Can you work these out from the model? Positions are in its coordinate system, mm. Face numbers are marked on the shaded views. A direction names the side the tool comes from. Round coordinates to 2 decimals unless told otherwise and drop trailing zeros. Write each loop counter-clockwise with the first axis right and the second up, starting at its lowest first coordinate (ties: lowest second). Pieces come first, ordered by that corner, then holes. Notation, with made-up numbers: (73, -13.75) - (110, -13.75) arc R33 cw to (110, 20.25) - close; hole circle Ø4 at (-2.5, 13.5). An arc over 180 degrees is marked (long way). One line per item, written item: value. Start each with the question number.
(1) I want a section at A-A on z = -35. List the corners of the cut face in (x, y) for me (3 decimals).
(2) If I drill on L1, parallel to X at y = -6.85, z = -35 (3 decimals); L2, parallel to X at y = -8.75, z = -32; L3, parallel to Z at x = -17.5, y = -5, over which ranges is the centre line in solid material (lowest first)? Write a range as from..to.
(3) I'm going to push flat-ended pins straight in: pin 1 Ø8 at (x, z) = (11, -121.5) entering from +Y; pin 2 Ø2 at (x, y) = (-6.5, -1.5) entering from -Z; pin 3 Ø10 at (y, z) = (-3.5, -134.5) entering from -X; pin 4 Ø11 at (x, z) = (1, -119) entering from -Y. Where does each tip first touch, or does it pass through?
(4) I want a section at B-B on z = -49.95. List the corners of the cut face in (x, y) for me.
(5) I want a section at C-C on z = -95. List the corners of the cut face in (x, y) for me (3 decimals), plus the area to 3 significant figures.
(6) I want a section at D-D on x = 2. List the corners of the cut face in (y, z) for me.
(7) On a 3-axis mill with a long thin cutter (end or side, diameter ignored), from which of +Z, -Z, +X, -X, +Y, -Y can I reach the whole of each face in a straight line? I mean the marked faces 4 and 5. Say none if no direction works.
(8) Thinking about a two-plate mould opening in X: for the marked faces 1, 2 and 3, which applies, +X half, -X half, draft (parallel to the pull), parting line (faces both ways), or undercut?
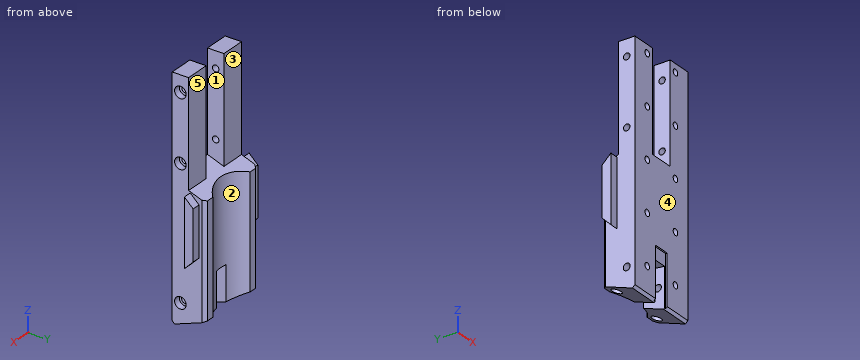
from build123d import *

# Parameters (mm, degrees)
SKETCH_1_W               = 63.621503831
SKETCH_1_H               = 9.95
EXTRUDE_1_DEPTH          = 22.5
CUT_EXTRUDE_START        = -7.55
CUT_EXTRUDE_1_DEPTH      = 15.1
CUT_EXTRUDE_2_DEPTH      = 145.249434495
CUT_EXTRUDE_2_DEPTH_BACK = 145.249434495
SKETCH_2_R               = 1.95
EXTRUDE_3_DEPTH          = 27.5
CUT_EXTRUDE_6_DEPTH      = 4.05
SKETCH_3_R               = 22.6
CUT_EXTRUDE_3_DEPTH      = 146.113401697
CUT_EXTRUDE_7_DEPTH      = 146.113401697
CUT_EXTRUDE_7_DEPTH_BACK = 146.113401697
SKETCH_10_R              = 2.1
SKETCH_11_W              = 39.483635772
SKETCH_11_H              = 6.923947262
CUT_EXTRUDE_8_DEPTH      = 5
CHAMFER_1_SIZE           = 2
SKETCH_4_R               = 3.5
CUT_EXTRUDE_4_DEPTH      = 4
SKETCH_12_R              = 3
CUT_EXTRUDE_9_DEPTH      = 3.1
CHAMFER_2_SIZE           = 2
CHAMFER_2_SIZE2          = 1.560412017
CHAMFER_2_EDGE_2_SIZE    = 2
CHAMFER_2_EDGE_2_SIZE2   = 1.560412017
SKETCH_13_R              = 1.925
CUT_EXTRUDE_10_DEPTH     = 5


# Read off the part's stored shape, not the designer's step: 컷-돌출1
with BuildPart() as part:
    # 스케치1 → 보스-돌출1 (new, symmetric)
    with BuildSketch(Plane(origin=(0, 0, 0), x_dir=(0, 0, -1), z_dir=(1, 0, 0))):
        with Locations((31.810751916, -4.975)):
            Rectangle(SKETCH_1_W, SKETCH_1_H)
        Polygon((142.136015324, -9.95), (63.621503831, -9.95), (63.621503831, 0), (67.243007662, 9.95), (134.893007662, 9.95), align=None)
        Polygon((63.621503831, -9.95), (63.621503831, 0), (60, -9.95), align=None)
    extrude(amount=EXTRUDE_1_DEPTH, both=True)

    # 컷-돌출1 outline → 컷-돌출1 (cut)
    with BuildSketch(Plane(origin=(0, 0, 0), x_dir=(0, 0, -1), z_dir=(1, 0, 0)).offset(CUT_EXTRUDE_START)):
        Polygon((60, -9.95), (63.621503831, 0), (0, 0), (0, -9.95), align=None)
    extrude(amount=CUT_EXTRUDE_1_DEPTH, mode=Mode.SUBTRACT)

    # 스케치2 → 컷-돌출2 (cut, two sides: drawn at the far end of the back side and taken through both)
    with BuildSketch(Plane(origin=(0, 0, 0), x_dir=(0, 0, -1), z_dir=(1, 0, 0)).offset(-CUT_EXTRUDE_2_DEPTH_BACK)):
        with Locations((9.95, -5)):
            Circle(SKETCH_2_R)
        with Locations((49.95, -5)):
            Circle(SKETCH_2_R)
    extrude(amount=CUT_EXTRUDE_2_DEPTH + CUT_EXTRUDE_2_DEPTH_BACK, mode=Mode.SUBTRACT)

    # 스케치6 → 보스-돌출3 (add, symmetric)
    with BuildSketch(Plane(origin=(0, 0, 0), x_dir=(0, 0, -1), z_dir=(1, 0, 0))):
        Polygon((64.701480994, 1.014614629), (69.728626839, 6.30205348), (99.728626839, 6.30205348), (105.104415209, 1.014614629), align=None)
    extrude(amount=EXTRUDE_3_DEPTH, both=True)

    # 스케치9 → 컷-돌출6 (cut, symmetric)
    with BuildSketch(Plane(origin=(0, 0, 0), x_dir=(0, 0, -1), z_dir=(1, 0, 0))):
        Polygon((139.292204442, 9.95), (148.391731499, -9.95), (117.656886036, -9.95), (115.43958996, 9.95), align=None)
    extrude(amount=CUT_EXTRUDE_6_DEPTH, both=True, mode=Mode.SUBTRACT)

    # 스케치3 → 컷-돌출3 (cut, through all)
    with BuildSketch(Plane.XY):
        with Locations((0, 26)):
            Circle(SKETCH_3_R)
    extrude(amount=-CUT_EXTRUDE_3_DEPTH, mode=Mode.SUBTRACT)

    # 스케치10 → 컷-돌출7 (cut, two sides: drawn at the far end of the back side and taken through both)
    with BuildSketch(Plane(origin=(0, 0, 0), x_dir=(0, 0, -1), z_dir=(1, 0, 0)).offset(-CUT_EXTRUDE_7_DEPTH_BACK)):
        with Locations((128.602443504, -5)):
            Circle(SKETCH_10_R)
    extrude(amount=CUT_EXTRUDE_7_DEPTH + CUT_EXTRUDE_7_DEPTH_BACK, mode=Mode.SUBTRACT)

    # 스케치11 → 컷-돌출8 (cut, symmetric)
    with BuildSketch(Plane(origin=(0, 0, 0), x_dir=(0, 0, -1), z_dir=(1, 0, 0))):
        with Locations((129.741817886, -12.461973631)):
            Rectangle(SKETCH_11_W, SKETCH_11_H)
    extrude(amount=CUT_EXTRUDE_8_DEPTH, both=True, mode=Mode.SUBTRACT)

    # 모따기1
    chamfer_1_edges = [part.edges().sort_by_distance(p)[0] for p in [
        (22.5, 9.95, -101.068007662),
        (-22.5, 9.95, -101.068007662),
    ]]
    chamfer(chamfer_1_edges, length=CHAMFER_1_SIZE)

    # 스케치4 → 컷-돌출4 (cut)
    with BuildSketch(Plane(origin=(22.5, 0, 0), x_dir=(0, 0, -1), z_dir=(1, 0, 0))):
        with Locations((9.95, -5)):
            Circle(SKETCH_4_R)
        with Locations((49.95, -5)):
            Circle(SKETCH_4_R)
        with Locations((128.602443504, -5)):
            Circle(SKETCH_4_R)
    extrude(amount=-CUT_EXTRUDE_4_DEPTH, mode=Mode.SUBTRACT)

    # 스케치12 → 컷-돌출9 (cut)
    with BuildSketch(Plane(origin=(0, 44.517705875, -122.311391657), x_dir=(-1, 0, 0), z_dir=(0, 0.3420201433256732, -0.9396926207859068))):
        with Locations(Location((-17, -42, 0), (0, 0, 90))):
            Circle(SKETCH_12_R)
        with Locations(Location((17, -42, 0), (0, 0, 90))):
            Circle(SKETCH_12_R)
    extrude(amount=-CUT_EXTRUDE_9_DEPTH, mode=Mode.SUBTRACT)

    # 모따기2
    chamfer_2_edges = [part.edges().sort_by_distance(p)[0] for p in [
        (-13.75, -9.95, -142.136015324),
    ]]
    chamfer_2_side = [part.faces().sort_by_distance(p)[0] for p in [
        (0, -9.95, -74.847019357),
    ]]
    chamfer(chamfer_2_edges, length=CHAMFER_2_SIZE, length2=CHAMFER_2_SIZE2, reference=chamfer_2_side[0])

    # 모따기2 edge 2
    chamfer_2_edge_2_edges = [part.edges().sort_by_distance(p)[0] for p in [
        (13.75, -9.95, -142.136015324),
    ]]
    chamfer_2_edge_2_side = [part.faces().sort_by_distance(p)[0] for p in [
        (0, -9.95, -74.847019357),
    ]]
    chamfer(chamfer_2_edge_2_edges, length=CHAMFER_2_EDGE_2_SIZE, length2=CHAMFER_2_EDGE_2_SIZE2, reference=chamfer_2_edge_2_side[0])

    # 스케치13 → 컷-돌출10 (cut)
    with BuildSketch(Plane.XZ.offset(9.95)):
        with Locations(Location((12, -5, 0), (0, 0, 270))):
            Circle(SKETCH_13_R)
        with Locations(Location((12, -35, 0), (0, 0, 270))):
            Circle(SKETCH_13_R)
        with Locations(Location((12, -65, 0), (0, 0, 270))):
            Circle(SKETCH_13_R)
        with Locations(Location((-12, -65, 0), (0, 0, 90))):
            Circle(SKETCH_13_R)
        with Locations(Location((-12, -35, 0), (0, 0, 90))):
            Circle(SKETCH_13_R)
        with Locations(Location((-12, -5, 0), (0, 0, 90))):
            Circle(SKETCH_13_R)
        with Locations(Location((12, -95, 0), (0, 0, 270))):
            Circle(SKETCH_13_R)
        with Locations(Location((12, -125, 0), (0, 0, 270))):
            Circle(SKETCH_13_R)
        with Locations(Location((-12, -125, 0), (0, 0, 231.333825211))):
            Circle(SKETCH_13_R)
        with Locations(Location((-12, -95, 0), (0, 0, 90))):
            Circle(SKETCH_13_R)
    extrude(amount=-CUT_EXTRUDE_10_DEPTH, mode=Mode.SUBTRACT)


solid = part.part
Established:
1. outline: (-22.5, -9.95) - (-13.925, -9.95) - (-13.925, -4.95) - (-10.075, -4.95) - (-10.075, -9.95) - (-7.55, -9.95) - (-7.55, 0) - (-22.5, 0) - close; (7.55, -9.95) - (10.075, -9.95) - (10.075, -4.95) - (13.925, -4.95) - (13.925, -9.95) - (22.5, -9.95) - (22.5, 0) - (7.55, 0) - close
2. L1: -22.5..-13.925, -10.075..-7.55, 7.55..10.075, 13.925..22.5
2. L2: -22.5..-7.55, 7.55..22.5
2. L3: -140.33..-130.7, -126.5..-51.9, -48..-11.9, -8..0
3. pin 1: y = 9.1
3. pin 2: z = -139.42
3. pin 3: x = -22.5
3. pin 4: y = -9.95
4. outline: (-22.5, -9.95) - (-7.55, -9.95) - (-7.55, -6.95) - (-22.5, -6.95) - close; (-22.5, -3.05) - (-7.55, -3.05) - (-7.55, 0) - (-22.5, 0) - close; (7.55, -9.95) - (22.5, -9.95) - (22.5, -8.5) - (18.5, -8.5) - (18.5, -6.95) - (7.55, -6.95) - close; (7.55, -3.05) - (18.5, -3.05) - (18.5, -1.5) - (22.5, -1.5) - (22.5, 0) - (7.55, 0) - close
5. outline: (-27.5, 1.015) - (-22.5, 1.015) - (-22.5, -9.95) - (-13.925, -9.95) - (-13.925, -4.95) - (-10.075, -4.95) - (-10.075, -9.95) - (10.075, -9.95) - (10.075, -4.95) - (13.925, -4.95) - (13.925, -9.95) - (22.5, -9.95) - (22.5, 1.015) - (27.5, 1.015) - (27.5, 6.302) - (22.5, 6.302) - (22.5, 7.95) - (20.5, 9.95) - (15.911, 9.95) arc R22.6 cw to (-15.911, 9.95) - (-20.5, 9.95) - (-22.5, 7.95) - (-22.5, 6.302) - (-27.5, 6.302) - close
5. area: 762 mm2
6. outline: (-9.95, -110) - (-9, -110) - (-9, -117.55) - (3.49, -116.16) - (3.49, -64.89) - (-9.95, -60) - close
7. face 4: +Z, -Z, +X, -X, -Y
7. face 5: +Z, +X, -X, +Y
8. face 1: undercut
8. face 2: undercut
8. face 3: draft
